Geometry check sheet. Reference: the model listing, model coordinates, mm. A direction names the side the tool comes from. Round coordinates to 2 decimals unless told otherwise and drop trailing zeros. Order: outer loops, then holes, each group sorted by start corner. A loop starts at its lowest first (then second) coordinate and runs counter-clockwise, first axis right, second up.
(1) Cross-section at B-B on z = 6.5. Enter the section's corners in (x, y).
(2) Gauge pin test, flat ends, axial feed: P1, Ø12, axis at x = -2, z = 30, coming from the +Y side; P2, Ø8, axis at y = 13, z = 56, coming from the -X side; P3, Ø1.3, axis at x = 15, y = 7, coming from the +Z side. Record the tip position at first contact, or that the pin passes through.
(3) Draft check along X on faces 1 (the face through (19.25, 5, 3)), 2 (the face through (14.51, 4.93, -8.483)), 3 (the face through (15, 5, 21.5)). Enter one of: pulls with the +X half, pulls with the -X half, needs draft (parallel to the pull), parting line crosses it, or undercut.
(4) Cross-section at D-D on z = 60.5. Enter the section's corners in (x, y), and give its area (3 significant figures).
(5) Cross-section at C-C on x = -13.5. Enter the section's corners in (y, z), and give its area (3 significant figures).
(6) Cross-section at A-A on y = 1.75. Enter the section's corners in (x, z).
(7) Set-up check for faces 4 (the face through (-3.476, 12.153, 54.283)), 5 (the face through (18.39, 5.07, 20.6)): record each of +Z, -Z, +X, -X, +Y, -Y from which the full face is reachable in a straight line by a thin tool's end or side.
(8) Thickness scan on L1, parallel to Z at x = 14.25, y = 7; L2, parallel to Z at x = -14.25, y = 3; L3, parallel to Y at x = -16, z = 55. Record the ranges inside material, lowest first.
from build123d import *

# Parameters (mm, degrees)
SKETCH1_W             = 38.5
SKETCH1_H             = 22.75
BOSS_EXTRUDE1_DEPTH   = 10
F_4_0MM_DOWEL_HOLE1_D = 4
BOSS_EXTRUDE2_DEPTH   = 10
SKETCH5_R             = 11.2395
CUT_EXTRUDE1_DEPTH    = 1.8542
SKETCH6_R             = 6.223
BOSS_EXTRUDE3_DEPTH   = 8.128


with BuildPart() as part:
    # Sketch1 → Boss-Extrude1 (new body)
    with BuildSketch(Plane(origin=(0, 0, 0), x_dir=(1, 0, 0), z_dir=(0, 1, 0))):
        with Locations((0, -0.125)):
            Rectangle(SKETCH1_W, SKETCH1_H)
    extrude(amount=BOSS_EXTRUDE1_DEPTH)

    # Ø4.0mm Dowel Hole1 (through all)
    with Locations(Plane(origin=(0, 10, 0), x_dir=(1, 0, 0), z_dir=(0, 1, 0))):
        with Locations((14.25, 6.5), (-14.25, -6.5), (-14.25, 6.5), (14.25, -6.5)):
            Hole(F_4_0MM_DOWEL_HOLE1_D / 2)

    # Sketch4 → Boss-Extrude2 (add)
    with BuildSketch(Plane.XZ.offset(-10)):
        with BuildLine():
            Line((-19.25, 21.5), (-19.25, 11.5))
            Line((-19.25, 11.5), (19.25, 11.5))
            Line((19.25, 11.5), (19.25, 18.5))
            ThreePointArc((19.25, 18.5), (18.371320344, 20.621320344), (16.25, 21.5))
            Line((16.25, 21.5), (14.639608634, 21.5))
            ThreePointArc((14.639608634, 21.5), (12.558414619, 22.339298384), (11.641715787, 24.387579018))
            Line((11.641715787, 24.387579018), (10.25, 61.5))
            ThreePointArc((10.25, 61.5), (-3.75, 75.5), (-17.75, 61.5))
            Line((-17.75, 61.5), (-19.25, 21.5))
        make_face()
    extrude(amount=BOSS_EXTRUDE2_DEPTH)

    # Sketch5 → Cut-Extrude1 (cut)
    with BuildSketch(Plane(origin=(0, 10, 0), x_dir=(1, 0, 0), z_dir=(0, 1, 0))):
        with Locations(Location((-3.75, -60.5, 0), (0, 0, 270))):
            Circle(SKETCH5_R)
    extrude(amount=-CUT_EXTRUDE1_DEPTH, mode=Mode.SUBTRACT)

    # Sketch6 → Boss-Extrude3 (add)
    with BuildSketch(Plane(origin=(0, 8.1458, 0), x_dir=(1, 0, 0), z_dir=(0, 1, 0))):
        with Locations(Location((-3.75, -60.5, 0), (0, 0, 270))):
            Circle(SKETCH6_R)
    extrude(amount=BOSS_EXTRUDE3_DEPTH)


solid = part.part
Found:
1. outline: (-19.25, 0) - (-16.25, 0) - (-16.25, 10) - (-19.25, 10) - close; (-12.25, 0) - (12.25, 0) - (12.25, 10) - (-12.25, 10) - close; (16.25, 0) - (19.25, 0) - (19.25, 10) - (16.25, 10) - close
2. P1: stops at y = 10
2. P2: stops at x = -18.06
2. P3: stops at z = 21.51
3. face 1: pulls with the +X half
3. face 2: undercut
3. face 3: needs draft
4. outline: (-17.79, 0) - (10.29, 0) - (10.29, 10) - (7.49, 10) - (7.49, 8.15) - (2.47, 8.15) - (2.47, 16.27) - (-9.97, 16.27) - (-9.97, 8.15) - (-14.99, 8.15) - (-14.99, 10) - (-17.79, 10) - close
4. area: 340 mm2
5. outline: (0, -11.25) - (10, -11.25) - (10, -8.35) - (0, -8.35) - close; (0, -4.65) - (10, -4.65) - (10, 4.65) - (0, 4.65) - close; (0, 8.35) - (10, 8.35) - (10, 54.91) - (8.15, 54.91) - (8.15, 66.09) - (10, 66.09) - (10, 71.55) - (0, 71.55) - close
5. area: 733 mm2
6. outline: (-19.25, -11.25) - (19.25, -11.25) - (19.25, 18.5) arc R3 ccw to (16.25, 21.5) - (14.64, 21.5) arc R3 cw to (11.64, 24.39) - (10.25, 61.5) arc R14 ccw to (-17.75, 61.5) - (-19.25, 21.5) - close; hole circle Ø4 at (-14.25, -6.5); hole circle Ø4 at (-14.25, 6.5); hole circle Ø4 at (14.25, -6.5); hole circle Ø4 at (14.25, 6.5)
7. face 4: +Y
7. face 5: +Z, +X, +Y, -Y
8. L1: z = -11.25 to -8.5, -4.5 to 4.5, 8.5 to 21.53
8. L2: z = -11.25 to -8.5, -4.5 to 4.5, 8.5 to 70.76
8. L3: y = 0 to 10
